from build123d import *

# Parameters (mm, degrees)
SKETCH1_W               = 40
SKETCH1_H               = 40
SKETCH1_W_2             = 20.4
SKETCH1_H_2             = 20.4
BOSS_EXTRUDE1_DEPTH     = 80
SKETCH1_2_W             = 40
SKETCH1_2_H             = 40
SKETCH1_2_W_2           = 20.4
SKETCH1_2_H_2           = 20.4
BOSS_EXTRUDE2_DEPTH     = 40
CUT_EXTRUDE1_DEPTH      = 91.68671347
CUT_EXTRUDE1_DEPTH_BACK = 91.68671347
SKETCH2_R               = 2.75
SKETCH3_R               = 13.2
SKETCH3_R_2             = 5.75
CUT_EXTRUDE2_DEPTH      = 8.5
CUT_EXTRUDE3_START      = -31.5
SKETCH3_3_R             = 13.2
SKETCH3_3_R_2           = 5.75
CUT_EXTRUDE3_DEPTH      = 8.5
SKETCH3_4_R             = 5.75
CUT_EXTRUDE4_DEPTH      = 95.403601626
FILLET1_R               = 5
FILLET2_R               = 5


with BuildPart() as part:
    # Sketch1 → Boss-Extrude1 (new body)
    with BuildSketch(Plane(origin=(0, 0, 0), x_dir=(1, 0, 0), z_dir=(0, 1, 0))):
        with Locations((10.2, 10.2)):
            Rectangle(SKETCH1_W, SKETCH1_H)
        with Locations((10.2, 10.2)):
            Rectangle(SKETCH1_W_2, SKETCH1_H_2, mode=Mode.SUBTRACT)
    extrude(amount=BOSS_EXTRUDE1_DEPTH)

    # Sketch1<2> → Boss-Extrude2 (add)
    # profile 1 of 2: a face of its own
    with BuildSketch(Plane(origin=(0, 0, 0), x_dir=(1, 0, 0), z_dir=(0, 1, 0))):
        with Locations((10.2, 10.2)):
            Rectangle(SKETCH1_2_W, SKETCH1_2_H)
        with Locations((10.2, 10.2)):
            Rectangle(SKETCH1_2_W_2, SKETCH1_2_H_2, mode=Mode.SUBTRACT)
    # profile 2 of 2: a face of its own
    with BuildSketch(Plane(origin=(0, 0, 0), x_dir=(1, 0, 0), z_dir=(0, 1, 0))):
        with Locations((10.2, 10.2)):
            Rectangle(SKETCH1_2_W_2, SKETCH1_2_H_2)
    extrude(amount=-BOSS_EXTRUDE2_DEPTH)

    # Sketch2 → Cut-Extrude1 (cut, two sides: drawn at the far end of the back side and taken through both)
    with BuildSketch(Plane(origin=(0, 0, 0), x_dir=(-1, 0, 0), z_dir=(0, 0, -1)).offset(-CUT_EXTRUDE1_DEPTH_BACK)):
        with Locations((-10.2, 15)):
            Circle(SKETCH2_R)
        with Locations((-10.2, 65)):
            Circle(SKETCH2_R)
    extrude(amount=CUT_EXTRUDE1_DEPTH + CUT_EXTRUDE1_DEPTH_BACK, mode=Mode.SUBTRACT)

    # Sketch3 → Cut-Extrude2 (cut)
    with BuildSketch(Plane.ZY.offset(9.8)):
        with Locations((-10.2, -20)):
            Circle(SKETCH3_R)
        with Locations((-10.2, -20)):
            Circle(SKETCH3_R_2, mode=Mode.SUBTRACT)
    extrude(amount=-CUT_EXTRUDE2_DEPTH, mode=Mode.SUBTRACT)

    # Sketch3<3> → Cut-Extrude3 (cut)
    with BuildSketch(Plane.ZY.offset(9.8).offset(CUT_EXTRUDE3_START)):
        with Locations((-10.2, -20)):
            Circle(SKETCH3_3_R)
        with Locations((-10.2, -20)):
            Circle(SKETCH3_3_R_2, mode=Mode.SUBTRACT)
    extrude(amount=-CUT_EXTRUDE3_DEPTH, mode=Mode.SUBTRACT)

    # Sketch3<4> → Cut-Extrude4 (cut, through all)
    with BuildSketch(Plane.ZY.offset(9.8)):
        with Locations((-10.2, -20)):
            Circle(SKETCH3_4_R)
    extrude(amount=-CUT_EXTRUDE4_DEPTH, mode=Mode.SUBTRACT)

    # Fillet1
    fillet1_edges = [part.edges().sort_by_distance(p)[0] for p in [
        (-9.8, 20, -30.2),
        (30.2, 20, -30.2),
        (30.2, 20, 9.8),
        (-9.8, 20, 9.8),
    ]]
    fillet(fillet1_edges, radius=FILLET1_R)

    # Fillet2
    fillet2_edges = [part.edges().sort_by_distance(p)[0] for p in [
        (-9.8, 80, -10.2),
        (10.2, 80, -30.2),
        (10.2, 80, 9.8),
        (30.2, 80, -10.2),
        (28.735533906, 80, -28.735533906),
        (28.735533906, 80, 8.335533906),
        (-8.335533906, 80, 8.335533906),
        (-8.335533906, 80, -28.735533906),
    ]]
    fillet(fillet2_edges, radius=FILLET2_R)


solid = part.part
Design review of the part built by this model. Coordinates are the model's own, in mm. A direction names the side the tool comes from. Round coordinates to 2 decimals unless told otherwise and drop trailing zeros. Write each loop counter-clockwise with the first axis right and the second up, starting at its lowest first coordinate (ties: lowest second). Pieces come first, ordered by that corner, then holes. Notation, with made-up numbers: M 68.5,-10.75 L 117.5,-10.75 A15 ccw 117.5,5.25 Z; hole C -10.75,80 d5. An arc over 180 degrees is marked long. One line per item, written item: value. Start each with the question number.
1. Clearance check with flat-ended pins moving along their axes: P1, Ø8, axis at y = -18, z = -4.5, coming from the +X side; P2, Ø3, axis at x = 3.5, z = -14.5, coming from the +Y side; P3, Ø24, axis at y = -20, z = -10.2, coming from the -X side. State where each tip first meets the part, or that it passes through.
2. To check wall thickness, follow probe 1 along X at (y, z) = (29, -18); probe 2 along Z at (x, y) = (4.5, 25.5); probe 3 along Y at (x, z) = (10, 2). State the ranges of each line that lie inside material, in increasing order. Write a range as from..to.
3. Take a section at D-D on x = 16. State the section outline as (y, z) points, then the cut area to 3 significant figures.
4. Take a section at B-B on y = -20. State the section outline as (x, z) points.
5. For faces 4 (the face through (21.7, -23, -5)), 5 (the face through (-1.3, -23, -5)), 6 (the face through (20.4, 39, -10)), 7 (the face through (10, -40, -10)), 8 (the face through (10.558, 17.727, 4.969)), list the 3-axis set-ups (+Z, -Z, +X, -X, +Y, -Y) from which the entire face can be reached by the end or side of a thin tool; tool diameter is ignored.
6. Take a section at C-C on z = -10.2. State the section outline as (x, y) points.
7. Draft analysis for pull direction Y (two halves, no side actions). For faces 1 (the face through (28.7, 16.7, -28.77)), 2 (the face through (25.89, -8.87, -3.1)), 3 (the face through (28.77, 78.5, -9.99)), state which applies: pulls with the +Y half, pulls with the -Y half, needs draft (parallel to the pull), parting line crosses it, or undercut.
8. Take a section at A-A on x = 10.2. State the section outline as (y, z) points, then the cut area to 3 significant figures.
Computed:
1. P1: stops at x = 21.7
1. P2: stops at y = 0
1. P3: stops at x = -1.3
2. probe 1: x = -9.8..0, 20.4..30.2
2. probe 2: z = -30.2..-20.4, 0..9.8
2. probe 3: y = -40..12.26, 17.74..62.26, 67.74..80
3. outline: M -40,-30.2 L 75,-30.2 A5 ccw 80,-25.2 L 80,-20.4 L 0,-20.4 L 0,0 L 80,0 L 80,4.8 A5 ccw 75,9.8 L -40,9.8 Z; hole C -20,-10.2 d11.5
3. area: 3,050 mm²
4. outline: M -9.8,-25.2 A5 ccw -4.8,-30.2 L 25.2,-30.2 A5 ccw 30.2,-25.2 L 30.2,-23.4 L 21.7,-23.4 L 21.7,-15.95 L -1.3,-15.95 L -1.3,-23.4 L -9.8,-23.4 Z; M -9.8,3 L -1.3,3 L -1.3,-4.45 L 21.7,-4.45 L 21.7,3 L 30.2,3 L 30.2,4.8 A5 ccw 25.2,9.8 L -4.8,9.8 A5 ccw -9.8,4.8 Z
5. face 4: +X
5. face 5: -X
5. face 6: +Y
5. face 7: +Z, -Z, +X, -X, -Y
5. face 8: +Z, -Z
6. outline: M -9.8,-40 L 30.2,-40 L 30.2,-33.2 L 21.7,-33.2 L 21.7,-25.75 L -1.3,-25.75 L -1.3,-33.2 L -9.8,-33.2 Z; M -9.8,-6.8 L -1.3,-6.8 L -1.3,-14.25 L 21.7,-14.25 L 21.7,-6.8 L 30.2,-6.8 L 30.2,75 A5 ccw 25.2,80 L 20.4,80 L 20.4,0 L 0,0 L 0,80 L -4.8,80 A5 ccw -9.8,75 Z
7. face 1: needs draft
7. face 2: undercut
7. face 3: pulls with the +Y half
8. outline: M -40,-30.2 L 12.25,-30.2 L 12.25,-20.4 L 0,-20.4 L 0,0 L 12.25,0 L 12.25,9.8 L -40,9.8 Z; M 17.75,-30.2 L 62.25,-30.2 L 62.25,-20.4 L 17.75,-20.4 Z; M 17.75,0 L 62.25,0 L 62.25,9.8 L 17.75,9.8 Z; M 67.75,-30.2 L 75,-30.2 A5 ccw 80,-25.2 L 80,-20.4 L 67.75,-20.4 Z; M 67.75,0 L 80,0 L 80,4.8 A5 ccw 75,9.8 L 67.75,9.8 Z; hole C -20,-10.2 d11.5
8. area: 2,840 mm²
